The figure shows three views and two pictorial views of one solid part (mm, origin at its lowest corner). Answer the questions. Give positions to 0.01 mm unless a question says otherwise; leave off trailing zeros. Write each loop counter-clockwise with the first axis right and the second up, starting at its lowest first coordinate (ties: lowest second). Pieces come first, ordered by that corner, then holes. Notation, with made-up numbers: M 13,46.5 L 53,46.5 A19 cw 53,81.5 Z; hole C -10,43.5 d7. An arc over 180 degrees is marked long. Return JSON: item names as keys, results as strings.
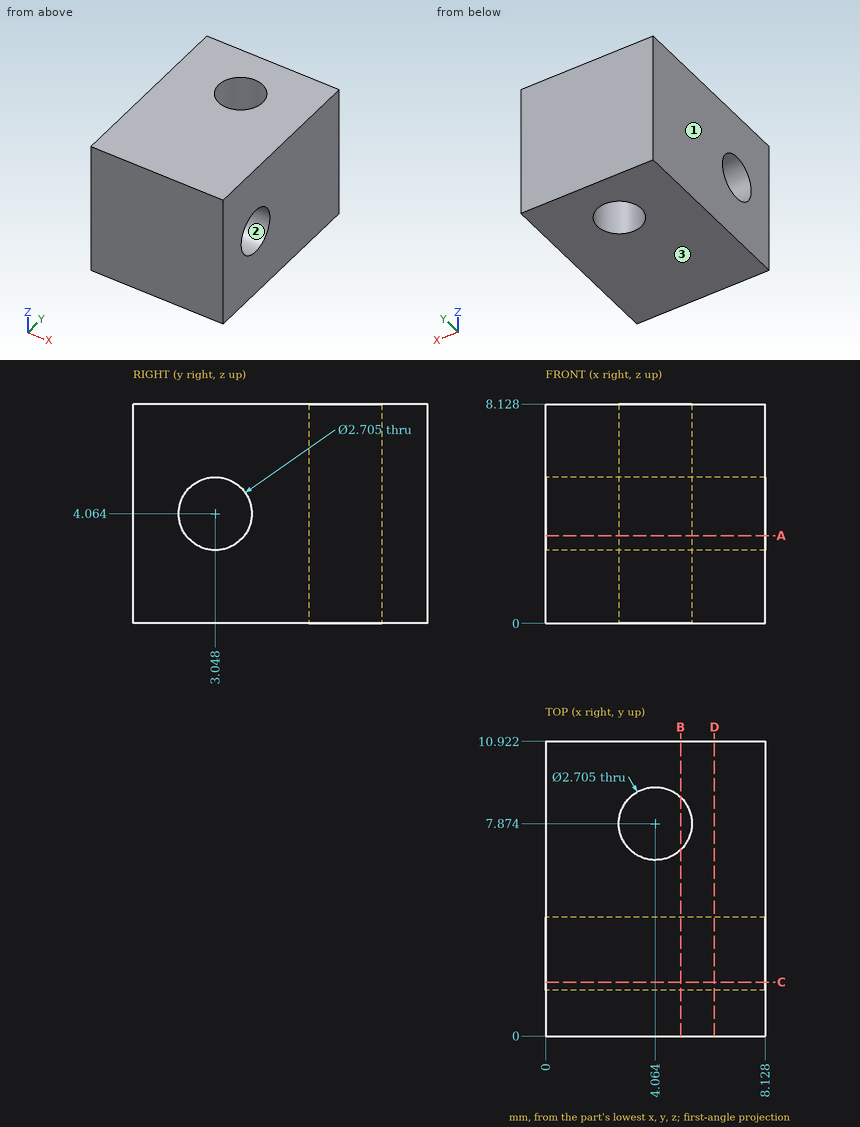
Item 1: A cutting plane is placed at C-C, the plane y = 2. Write down the section's boundary in (x, z), plus the area to 3 significant figures.
Geometry results:
{"outline": "M 0,0 L 8.13,0 L 8.13,3.21 L 0,3.21 Z; M 0,4.92 L 8.13,4.92 L 8.13,8.13 L 0,8.13 Z", "area": "52.2 mm2"}
Item 2: Given pin 1 Ø1.6 at (y, z) = (3.048, 4.064) entering from +X; pin 2 Ø4.5 at (x, y) = (4.064, 7.874) entering from -Z, each flat-ended and moving along its own axis, determine where each tip first touches the part or whether it passes through.
Geometry results:
{"pin 1": "passes through", "pin 2": "stops at z = 0"}
Item 3: A cutting plane is placed at A-A, the plane z = 3.25. Write down the section's boundary in (x, y) (1 decimal), plus the area to 3 significant figures.
Geometry results:
{"outline": "M 0,0 L 8.1,0 L 8.1,2 L 0,2 Z; M 0,4.1 L 8.1,4.1 L 8.1,10.9 L 0,10.9 Z; hole C 4.1,7.9 d2.7", "area": "65.5 mm2"}
Item 4: Determine the mould class of the marked faces 1, 2 and 3 for opening direction Z: +Z half, -Z half, draft (parallel to the pull), parting line (faces both ways), or undercut.
Geometry results:
{"face 1": "draft", "face 2": "undercut", "face 3": "-Z half"}
Item 5: Find the intervals of material crossed by line 1 (Y direction, x = 4, z = 1.75) (3 decimals); line 2 (Y direction, x = 3.5, z = 3) (1 decimal); line 3 (Z direction, x = 4.75, y = 3.5), in increasing order.
Geometry results:
{"line 1": "y = 0 to 6.523, 9.225 to 10.922", "line 2": "y = 0 to 2.2, 3.9 to 6.6, 9.1 to 10.9", "line 3": "z = 0 to 2.79, 5.34 to 8.13"}
Item 6: A cutting plane is placed at D-D, the plane x = 6.25. Write down the section's boundary in (y, z) (1 decimal), plus the area to 3 significant figures.
Geometry results:
{"outline": "M 0,0 L 10.9,0 L 10.9,8.1 L 0,8.1 Z; hole C 3,4.1 d2.7", "area": "83.0 mm2"}
Item 7: A cutting plane is placed at B-B, the plane x = 5. Write down the section's boundary in (y, z) (1 decimal).
Geometry results:
{"outline": "M 0,0 L 6.9,0 L 6.9,8.1 L 0,8.1 Z; M 8.9,0 L 10.9,0 L 10.9,8.1 L 8.9,8.1 Z; hole C 3,4.1 d2.7"}
